from build123d import *

# Parameters (mm, degrees)
SKETCH2_R           = 2
BOSS_EXTRUDE1_DEPTH = 5
FILLET1_START       = -1
FILLET1_DEPTH       = 7
FILLET1_2_DEPTH     = 5
BOSS_EXTRUDE2_DEPTH = 8.8
SKETCH4_W           = 22
SKETCH4_H           = 2.3
CUT_EXTRUDE1_DEPTH  = 46
SKETCH5_W           = 2
SKETCH5_H           = 2.3
CUT_EXTRUDE2_DEPTH  = 20
FILLET2_R           = 5
FILLET3_R           = 2.5


with BuildPart() as part:
    # Sketch2 → Boss-Extrude1 (new body)
    with BuildSketch(Plane(origin=(0, 0, 0), x_dir=(1, 0, 0), z_dir=(0, 1, 0))):
        Polygon((5, 12.5), (25, 12.5), (25, -17.5), (5, -17.5), (5, -27.5), (-5, -27.5), (-5, -17.5), (-25, -17.5), (-25, 12.5), (-5, 12.5), (-5, 22.5), (5, 22.5), align=None)
        with Locations(Location((0, 17.5, 0), (0, 0, 270))):
            Circle(SKETCH2_R, mode=Mode.SUBTRACT)
        with Locations(Location((0, -22.5, 0), (0, 0, 90))):
            Circle(SKETCH2_R, mode=Mode.SUBTRACT)
    extrude(amount=BOSS_EXTRUDE1_DEPTH)

    # Fillet1: read off the stored shape, not the designer's step
    # Fillet1 outline → Fillet1 (cut)
    with BuildSketch(Plane(origin=(0, 0, 0), x_dir=(1, 0, 0), z_dir=(0, 1, 0)).offset(FILLET1_START)):
        with BuildLine():
            ThreePointArc((5, -22.5), (3.535533906, -26.035533906), (0, -27.5))
            Line((0, -27.5), (5, -27.5))
            Line((5, -27.5), (5, -22.5))
        make_face()
        with BuildLine():
            ThreePointArc((0, -27.5), (-3.535533906, -26.035533906), (-5, -22.5))
            Line((-5, -22.5), (-5, -27.5))
            Line((-5, -27.5), (0, -27.5))
        make_face()
        with BuildLine():
            ThreePointArc((-5, 17.5), (-3.535533906, 21.035533906), (0, 22.5))
            Line((0, 22.5), (-5, 22.5))
            Line((-5, 22.5), (-5, 17.5))
        make_face()
        with BuildLine():
            ThreePointArc((0, 22.5), (3.535533906, 21.035533906), (5, 17.5))
            Line((5, 17.5), (5, 22.5))
            Line((5, 22.5), (0, 22.5))
        make_face()
    extrude(amount=FILLET1_DEPTH, mode=Mode.SUBTRACT)

    # Fillet1 2 outline → Fillet1 2 (add)
    with BuildSketch(Plane(origin=(0, 0, 0), x_dir=(1, 0, 0), z_dir=(0, 1, 0))):
        with BuildLine():
            Line((5, -17.5), (5, -22.5))
            ThreePointArc((5, -22.5), (6.464466094, -18.964466094), (10, -17.5))
            Line((10, -17.5), (5, -17.5))
        make_face()
        with BuildLine():
            ThreePointArc((-10, -17.5), (-6.464466094, -18.964466094), (-5, -22.5))
            Line((-5, -22.5), (-5, -17.5))
            Line((-5, -17.5), (-10, -17.5))
        make_face()
        with BuildLine():
            Line((-5, 12.5), (-5, 17.5))
            ThreePointArc((-5, 17.5), (-6.464466094, 13.964466094), (-10, 12.5))
            Line((-10, 12.5), (-5, 12.5))
        make_face()
        with BuildLine():
            ThreePointArc((10, 12.5), (6.464466094, 13.964466094), (5, 17.5))
            Line((5, 17.5), (5, 12.5))
            Line((5, 12.5), (10, 12.5))
        make_face()
    extrude(amount=FILLET1_2_DEPTH)

    # Sketch3 → Boss-Extrude2 (add)
    with BuildSketch(Plane(origin=(0, 5, 0), x_dir=(1, 0, 0), z_dir=(0, 1, 0))):
        Polygon((-25, -11.5), (-25, -17.5), (25, -17.5), (25, 12.5), (-25, 12.5), (-25, 6.5), (19, 6.5), (19, -11.5), align=None)
    extrude(amount=BOSS_EXTRUDE2_DEPTH)

    # Sketch4 → Cut-Extrude1 (cut)
    with BuildSketch(Plane.ZY.offset(25)):
        with Locations((2.5, 12.65)):
            Rectangle(SKETCH4_W, SKETCH4_H)
    extrude(amount=-CUT_EXTRUDE1_DEPTH, mode=Mode.SUBTRACT)

    # Sketch5 → Cut-Extrude2 (cut)
    with BuildSketch(Plane.ZY.offset(25)):
        with Locations((-9.5, 12.65)):
            Rectangle(SKETCH5_W, SKETCH5_H)
        with Locations((14.5, 12.65)):
            Rectangle(SKETCH5_W, SKETCH5_H)
    extrude(amount=-CUT_EXTRUDE2_DEPTH, mode=Mode.SUBTRACT)

    # Fillet2
    fillet2_edges = [part.edges().sort_by_distance(p)[0] for p in [
        (25, 6.9, 17.5),
        (25, 6.9, -12.5),
    ]]
    fillet(fillet2_edges, radius=FILLET2_R)

    # Fillet3
    fillet3_edges = [part.edges().sort_by_distance(p)[0] for p in [
        (-25, 8.25, 11.5),
        (-25, 8.25, -6.5),
        (-25, 5, 2.5),
        (0, 5, 17.5),
        (0, 5, -12.5),
    ]]
    fillet(fillet3_edges, radius=FILLET3_R)


solid = part.part
Geometry: final body of the model. Coordinates: model frame, mm. A direction names the side the tool comes from. Give positions to 0.01 mm unless a question says otherwise; leave off trailing zeros. Order: outer loops, then holes, each group sorted by start corner. A loop starts at its lowest first (then second) coordinate and runs counter-clockwise, first axis right, second up. Notation, with made-up numbers: (-18.75, 44.5) -> (-11.75, 44.5) arc R11 cw to (-11.75, 53.5) -> close; hole circle Ø11 at (-27.5, -12). An arc over 180 degrees is marked (long way). Answer as a JSON object with one key per item and string values.
Q1. Material intervals for probe 1 along Z at (x, y) = (-15, 12.5); probe 2 along X at (y, z) = (3, -17.5); probe 3 along Z at (x, y) = (-3.5, 10), sorted ascending.
Entries:
{"probe 1": "z = -12.5 to -10.5, 15.5 to 17.5", "probe 2": "x = -5 to -2, 2 to 5", "probe 3": "z = -12.5 to -6.5, 11.5 to 17.5"}
Q2. Section D-D (x = -3.5). Output: boundary loops of the cut face in (y, z), plus the area to 3 significant figures.
Entries:
{"outline": "(0, -21.07) -> (5, -21.07) -> (5, -15) arc R2.5 cw to (7.5, -12.5) -> (13.8, -12.5) -> (13.8, -8.5) -> (11.5, -8.5) -> (11.5, -6.5) -> (5, -6.5) -> (5, 11.5) -> (11.5, 11.5) -> (11.5, 13.5) -> (13.8, 13.5) -> (13.8, 17.5) -> (7.5, 17.5) arc R2.5 cw to (5, 20) -> (5, 26.07) -> (0, 26.07) -> close", "area": "335 mm^2"}
Q3. Section B-B (z = 4). Output: boundary loops of the cut face in (x, y), plus the area to 3 significant figures.
Entries:
{"outline": "(-25, 0) -> (25, 0) -> (25, 13.8) -> (21, 13.8) -> (21, 11.5) -> (19, 11.5) -> (19, 5) -> (-22.5, 5) arc R2.5 ccw to (-25, 2.5) -> close", "area": "297 mm^2"}
Q4. Section A-A (x = -16.5). Output: boundary loops of the cut face in (y, z).
Entries:
{"outline": "(0, -12.5) -> (13.8, -12.5) -> (13.8, -10.5) -> (11.5, -10.5) -> (11.5, -6.5) -> (5, -6.5) -> (5, 11.5) -> (11.5, 11.5) -> (11.5, 15.5) -> (13.8, 15.5) -> (13.8, 17.5) -> (0, 17.5) -> close"}
Q5. Access query for faces 4 (the flat face through (-3, 8, -12.5)), 5 (the flat face through (-3, 8, 17.5)), 6 (the flat face through (21, 13, 2)). Directions: +Z, -Z, +X, -X, +Y, -Y. A direction counts if a zero-diameter tool reaches every point of the face in a straight line with its end or side. Return the directions, or none.
Entries:
{"face 4": "-Z, +Y", "face 5": "+Z, +Y", "face 6": "-X, +Y"}
Q6. Section C-C (z = -11.5). Output: boundary loops of the cut face in (x, y), plus the area to 3 significant figures.
Entries:
{"outline": "(-25, 0) -> (23, 0) -> (23, 13.8) -> (-25, 13.8) -> close", "area": "662 mm^2"}
Q7. First-contact query: pin 1 (4 mm diameter, centred on x = 0.5, z = 25.5, fed in from +Y); pin 2 (2.5 mm diameter, centred on x = -12, y = 12.5, fed in from +Z); pin 3 (1 mm diameter, centred on y = 1.5, z = 13.5, fed in from +X). Flat tips, straight axial feed; report the tip coordinate or a pass-through.
Entries:
{"pin 1": "stops at y = 5", "pin 2": "stops at z = 17.5", "pin 3": "stops at x = 24.97"}
Q8. Draft query along X for faces 1 (the cylindrical face through (-1.2, 2.5, -19.1)), 2 (the flat face through (-5, 13, -10)), 3 (the flat face through (-1, 8, 11.5)). Return one class per face: released by +X, released by -X, zero draft, split by the parting line, or undercut.
Entries:
{"face 1": "undercut", "face 2": "released by -X", "face 3": "zero draft"}
